The listing builds one solid part. Answer for the finished solid, in the listing's coordinates (mm). A direction names the side the tool comes from. Round coordinates to 2 decimals unless told otherwise and drop trailing zeros. Write each loop counter-clockwise with the first axis right and the second up, starting at its lowest first coordinate (ties: lowest second). Pieces come first, ordered by that corner, then holes.
from build123d import *

# Parameters (mm, degrees)
BOSS_EXTRUDE1_DEPTH = 10
BOSS_EXTRUDE2_DEPTH = 2


with BuildPart() as part:
    # Sketch1 → Boss-Extrude1 (new body)
    with BuildSketch(Plane(origin=(0, 0, 0), x_dir=(0, 0, -1), z_dir=(1, 0, 0))):
        Polygon((-3.774433469, 39.035588244), (-3.774433469, 9.358035215), (-3.774433469, 7.792183966), (-3.774433469, -19.326020697), (-3.774433469, -21.674922387), (-3.774433469, -43.604639285), (-35.757790758, -43.604639285), (-38.060598591, -45.851882357), (-2.255261006, -45.851882357), (-2.255261006, 30.924278392), (-2.255261006, 34.77223015), (-2.255261006, 40.341171907), (-38.060598591, 40.341171907), (-35.757790758, 39.035588244), align=None)
        Polygon((-3.774433469, 9.358035215), (-35.757790758, 29.614700037), (-35.757790758, 27.080766413), (-3.774433469, 7.792183966), align=None)
        Polygon((-3.774433469, -21.674922387), (-3.774433469, -19.326020697), (-35.757790758, -5.486543586), (-35.757790758, -8.33500588), align=None)
    boss_extrude1 = extrude(amount=BOSS_EXTRUDE1_DEPTH)

    # Sketch1_4 → Boss-Extrude2 (add)
    with BuildSketch(Plane(origin=(0, 0, 0), x_dir=(0, 0, -1), z_dir=(1, 0, 0))):
        Polygon((-3.774433469, -21.674922387), (-3.774433469, -19.326020697), (-35.757790758, -5.486543586), (-35.757790758, -8.33500588), align=None)
        Polygon((-3.774433469, 9.358035215), (-35.757790758, 29.614700037), (-35.757790758, 27.080766413), (-3.774433469, 7.792183966), align=None)
        Polygon((-38.060598591, -45.851882357), (-35.757790758, -43.604639285), (-3.774433469, -43.604639285), (-3.774433469, 39.035588244), (-35.757790758, 39.035588244), (-38.060598591, 40.341171907), (-2.255261006, 40.341171907), (-2.255261006, -45.851882357), align=None)
        Polygon((4.824416605, 33.833827141), (-2.255261006, 34.77223015), (-2.255261006, 30.924278392), (1.146733549, 29.614700037), (2.396539842, 22.331937706), (6.798273933, 22.331937706), align=None)
        Polygon((-35.757790758, 27.080766413), (-35.757790758, 29.614700037), (-3.774433469, 9.358035215), (-3.774433469, 39.035588244), (-35.757790758, 39.035588244), (-38.060598591, 40.341171907), (-38.060598591, -45.851882357), (-35.757790758, -43.604639285), (-3.774433469, -43.604639285), (-3.774433469, -21.674922387), (-35.757790758, -8.33500588), (-35.757790758, -5.486543586), (-3.774433469, -19.326020697), (-3.774433469, 7.792183966), align=None)
    boss_extrude2 = extrude(amount=-BOSS_EXTRUDE2_DEPTH)

    # Mirror1: Boss-Extrude1, Boss-Extrude2 across plane
    add(boss_extrude1.mirror(Plane(origin=(10, 0, 0), x_dir=(0, 0, 1), z_dir=(1, 0, 0))))
    add(boss_extrude2.mirror(Plane(origin=(10, 0, 0), x_dir=(0, 0, 1), z_dir=(1, 0, 0))))


solid = part.part
1. Section B-B on z = 25.5 is taken. Determine the outline of the cut face in (x, y).
Geometry says:
outline: (-2, -45.85) - (22, -45.85) - (22, 40.34) - (-2, 40.34) - close; hole (0, -43.6) - (20, -43.6) - (20, -12.61) - (0, -12.61) - close; hole (0, -9.93) - (20, -9.93) - (20, 20.89) - (0, 20.89) - close; hole (0, 23.12) - (20, 23.12) - (20, 39.04) - (0, 39.04) - close
2. For a pull along X with two mould halves and no side action, classify faces 5 (the face through (-0.986, 26.024, -1.763)), 6 (the face through (-2, -2, 21)), 7 (the face through (10, -7, 35.758)) as released by +X, released by -X, zero draft, split by the parting line, or undercut.
Geometry says:
face 5: zero draft
face 6: released by -X
face 7: undercut
3. Section C-C on x = 10.25 is taken. Determine the outline of the cut face in (y, z) (3 decimals).
Geometry says:
outline: (-45.852, 2.255) - (40.341, 2.255) - (40.341, 38.061) - (39.036, 35.758) - (39.036, 3.774) - (9.358, 3.774) - (29.615, 35.758) - (27.081, 35.758) - (7.792, 3.774) - (-19.326, 3.774) - (-5.487, 35.758) - (-8.335, 35.758) - (-21.675, 3.774) - (-43.605, 3.774) - (-43.605, 35.758) - (-45.852, 38.061) - close
4. Given pin 1 (3 mm diameter, centred on x = 14, y = 29, fed in from +Z); pin 2 (0.6 mm diameter, centred on x = -1, z = -4, fed in from -Y); pin 3 (2.5 mm diameter, centred on y = 27, z = -1, fed in from +X); pin 4 (1.5 mm diameter, centred on x = 2.5, y = -28.5, fed in from +Z), each flat-ended and moving along its own axis, determine where each tip first touches the part or whether it passes through.
Geometry says:
pin 1: stops at z = 35.76
pin 2: stops at y = 22.33
pin 3: stops at x = 22
pin 4: stops at z = 3.77
5. Straight lines are drawn through the part: line 1 along Y through (x, z) = (14, 13); line 2 along X through (y, z) = (23, 20); line 3 along Y through (x, z) = (15.25, 26). For each, find the intervals that lie inside material, in ascending order.
Geometry says:
line 1: y = -45.85 to -43.6, -17.83 to -15.33, 13.36 to 15.2, 39.04 to 40.34
line 2: x = -2 to 0, 20 to 22
line 3: y = -45.85 to -43.6, -12.4 to -9.71, 21.2 to 23.43, 39.04 to 40.34
6. A tool of negligible diameter and unlimited length cuts with its end or side. For faces 1 (the face through (10, 24, 3.774)), 2 (the face through (0, 29, -2)), 3 (the face through (10.14, -44.71, 36.89)), 4 (the face through (20.99, 30.28, 0.58)), from which of +Z, -Z, +X, -X, +Y, -Y can it reach the whole face along a straight path? Write none if from no direction.
Geometry says:
face 1: none
face 2: -Z, +Y, -Y
face 3: +Z
face 4: +X, -X, -Y
7. Section A-A on y = -35 is taken. Determine the outline of the cut face in (x, z).
Geometry says:
outline: (-2, 2.26) - (22, 2.26) - (22, 38.06) - (20, 38.06) - (20, 3.77) - (0, 3.77) - (0, 38.06) - (-2, 38.06) - close
8. Section D-D on y = -13.5 is taken. Determine the outline of the cut face in (x, z), plus the area to 3 significant figures.
Geometry says:
outline: (-2, 2.26) - (22, 2.26) - (22, 38.06) - (20, 38.06) - (20, 23.37) - (0, 23.37) - (0, 38.06) - (-2, 38.06) - close; hole (0, 3.77) - (20, 3.77) - (20, 17.24) - (0, 17.24) - close
area: 296 mm2
